Design review of the part built by this model. Coordinates are the model's own, in mm. A direction names the side the tool comes from. Give positions to 0.01 mm unless a question says otherwise; leave off trailing zeros. Write each loop counter-clockwise with the first axis right and the second up, starting at its lowest first coordinate (ties: lowest second). Pieces come first, ordered by that corner, then holes. Notation, with made-up numbers: (39, -15.5) -> (82, -15.5) arc R21 ccw to (82, -0.5) -> close; hole circle Ø4 at (11.5, -13.5). An arc over 180 degrees is marked (long way). Answer as a JSON object with one key per item and string values.
```python
from build123d import *

# Parameters (mm, degrees)
F0_R     = 5.15
F1_DEPTH = 3
F0_R_2   = 7
F2_DEPTH = 5.26


with BuildPart() as f1:
    # F0 (on Top) → F1 (new body)
    with BuildSketch(Plane.XY):
        Circle(F0_R)
        with BuildLine():
            ThreePointArc((-1.7, 3.116488), (3.55, 0), (-1.7, -3.116488))
            Line((-1.7, -3.116488), (-1.7, 3.116488))
        make_face(mode=Mode.SUBTRACT)
    extrude(amount=F1_DEPTH)

    # F0 (on Top) → F2 (join)
    with BuildSketch(Plane.XY):
        Circle(F0_R_2)
        Circle(F0_R, mode=Mode.SUBTRACT)
    extrude(amount=F2_DEPTH)


solid = f1.part
```
(1) We need section D-D, the plane y = -4.75. State the section outline as (x, z) points, then the cut area to 3 significant figures.
Here are the results:
{"outline": "(-5.14, 0) -> (5.14, 0) -> (5.14, 5.26) -> (1.99, 5.26) -> (1.99, 3) -> (-1.99, 3) -> (-1.99, 5.26) -> (-5.14, 5.26) -> close", "area": "45.1 mm²"}
(2) For line 1 along Y through (x, z) = (0, 1.6); line 2 along Y through (x, z) = (0, 4.7); line 3 along Z through (x, y) = (-2.25, 3.75), list the stretches that pass through material, from the lowest coordinate up.
Here are the results:
{"line 1": "y = -7 to -3.55, 3.55 to 7", "line 2": "y = -7 to -5.15, 5.15 to 7", "line 3": "z = 0 to 3"}
(3) We need section A-A, the plane x = 0. State the section outline as (y, z) points, then the cut area to 3 significant figures.
Here are the results:
{"outline": "(-7, 0) -> (-3.55, 0) -> (-3.55, 3) -> (-5.15, 3) -> (-5.15, 5.26) -> (-7, 5.26) -> close; (3.55, 0) -> (7, 0) -> (7, 5.26) -> (5.15, 5.26) -> (5.15, 3) -> (3.55, 3) -> close", "area": "29.1 mm²"}
(4) The part is to be moulded in two halves that separate along Y. For faces 1 (the flat face through (-1.7, 0, 1)), 2 (the flat face through (-3, 0, 0)), 3 (the cylindrical face through (6.466, -2.681, 2.593)), 4 (the flat face through (-2, 0, 3)), say which applies: +Y half, -Y half, draft (parallel to the pull), parting line (faces both ways), or undercut.
Here are the results:
{"face 1": "undercut", "face 2": "draft", "face 3": "parting line", "face 4": "undercut"}
(5) We need section B-B, the plane y = 0. State the section outline as (x, z) points.
Here are the results:
{"outline": "(-7, 0) -> (-1.7, 0) -> (-1.7, 3) -> (-5.15, 3) -> (-5.15, 5.26) -> (-7, 5.26) -> close; (3.55, 0) -> (7, 0) -> (7, 5.26) -> (5.15, 5.26) -> (5.15, 3) -> (3.55, 3) -> close"}
(6) We need section C-C, the plane z = 3.3. State the section outline as (x, y) points, then the cut area to 3 significant figures.
Here are the results:
{"outline": "circle Ø14 at (0, 0); hole circle Ø10.3 at (0, 0)", "area": "70.6 mm²"}
(7) Clearance check with flat-ended pins moving along their axes: pin 1 (2 mm diameter, centred on y = 4.5, z = 3, fed in from -X); pin 2 (2 mm diameter, centred on y = -2.5, z = 3.5, fed in from +X); pin 3 (3 mm diameter, centred on x = -1, y = -1, fed in from +Z). State where each tip first meets the part, or that it passes through.
Here are the results:
{"pin 1": "stops at x = -6.06", "pin 2": "stops at x = 6.84", "pin 3": "stops at z = 3"}
(8) For faces 5 (the cylindrical face through (4.91, 1.55, 4.11)), 6 (the flat face through (-4, 4, 5.26)), list the 3-axis set-ups (+Z, -Z, +X, -X, +Y, -Y) from which the entire face can be reached by the end or side of a thin tool; tool diameter is ignored.
Here are the results:
{"face 5": "+Z", "face 6": "+Z, +X, -X, +Y, -Y"}
